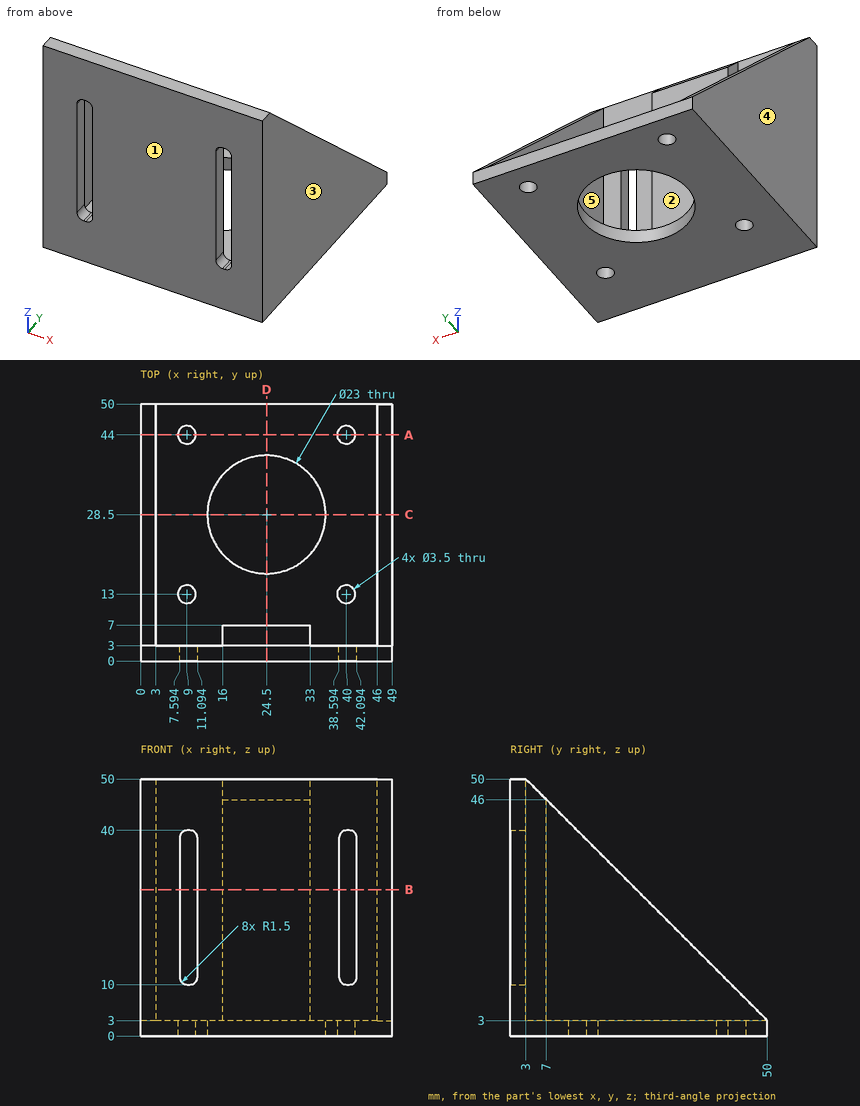
Part print with two shaded views. Sizes in mm from the minimum x, y, z corner. A direction names the side the tool comes from. Give positions to 0.01 mm unless a question says otherwise; leave off trailing zeros. Loops run counter-clockwise (first coordinate to the right, second up) from the corner with the lowest first, then second, coordinate; pieces in that order, holes last. Notation, with made-up numbers: (-22.75, 82) - (4.25, 82) arc R25 cw to (4.25, 111) - close; hole circle Ø1 at (63.25, -24.75). An arc over 180 degrees is marked (long way). Put each result on its own line as item: value.
Q1. Slice it at C-C (y = 28.5). Give the cut face in (x, z), plus the area to 3 significant figures.
Filled in:
outline: (0, 0) - (13, 0) - (13, 3) - (3, 3) - (3, 24.5) - (0, 24.5) - close; (36, 0) - (49, 0) - (49, 24.5) - (46, 24.5) - (46, 3) - (36, 3) - close
area: 207 mm²
Q2. Slice it at D-D (x = 24.5). Give the cut face in (y, z).
Filled in:
outline: (0, 0) - (17, 0) - (17, 3) - (7, 3) - (7, 46) - (3, 50) - (0, 50) - close; (40, 0) - (50, 0) - (50, 3) - (40, 3) - close
Q3. Probe line 1 along Y through (x, z) = (40, 1.35); line 2 along X through (y, z) = (39.5, 7); line 3 along X through (y, z) = (28, 1). List the from-to ranges inside material, lowest first.
Filled in:
line 1: y = 0 to 11.25, 14.75 to 42.25, 45.75 to 50
line 2: x = 0 to 3, 46 to 49
line 3: x = 0 to 13.01, 35.99 to 49
Q4. Flat gauge pins, fed straight in: pin 1 (2 mm diameter, centred on x = 16, y = 32, fed in from +Z); pin 2 (4 mm diameter, centred on x = 12, z = 28.5, fed in from +Y); pin 3 (14.5 mm diameter, centred on x = 36.5, z = 35, fed in from +Y); pin 4 (6 mm diameter, centred on x = 8.5, y = 11.5, fed in from +Z). Where does each tip first touch, or does it go through?
Filled in:
pin 1: passes through
pin 2: stops at y = 3
pin 3: stops at y = 7
pin 4: stops at z = 3
Q5. Slice it at A-A (y = 44). Give the cut face in (x, z), plus the area to 3 significant figures.
Filled in:
outline: (0, 0) - (7.25, 0) - (7.25, 3) - (3, 3) - (3, 9) - (0, 9) - close; (10.75, 0) - (38.25, 0) - (38.25, 3) - (10.75, 3) - close; (41.75, 0) - (49, 0) - (49, 9) - (46, 9) - (46, 3) - (41.75, 3) - close
area: 162 mm²
Q6. Tool access for the marked faces 4 and 5: list every direction of +Z, -Z, +X, -X, +Y, -Y with a clear straight run to the whole face (end or side of a thin tool).
Filled in:
face 4: +Z, -Z, -X, +Y, -Y
face 5: +Z, +Y
Q7. Slice it at B-B (z = 28.5). Give the cut face in (x, y) (1 decimal).
Filled in:
outline: (0, 0) - (7.6, 0) - (7.6, 3) - (3, 3) - (3, 24.5) - (0, 24.5) - close; (11.1, 0) - (38.6, 0) - (38.6, 3) - (33, 3) - (33, 7) - (16, 7) - (16, 3) - (11.1, 3) - close; (42.1, 0) - (49, 0) - (49, 24.5) - (46, 24.5) - (46, 3) - (42.1, 3) - close
Q8. Mould opens along X. For the marked faces 1, 2 and 3 say: pulls with the +X half, pulls with the -X half, needs draft (parallel to the pull), parting line crosses it, or undercut.
Filled in:
face 1: needs draft
face 2: undercut
face 3: pulls with the +X half
